Check sheet for the modelled part. Datum: model origin and axes. Units: mm. A direction names the side the tool comes from. Coordinates: 2 decimals unless noted, no trailing zeros. Loops run counter-clockwise (first coordinate to the right, second up) from the corner with the lowest first, then second, coordinate; pieces in that order, holes last.
Autodesk Inventor part; units mm, degrees
ref_plane "YZ Plane" through (0, 0, 0) normal (1, 0, 0) x (0, 1, 0)
ref_plane "XZ Plane" through (0, 0, 0) normal (0, 1, 0) x (-1, 0, 0)
ref_plane "XY Plane" through (0, 0, 0) normal (0, 0, 1) x (1, 0, 0)
sketch "Sketch1" plane through (0, 0, 0) normal (0, 1, 0) x (-1, 0, 0)
  circle A0 centre (0, 0) radius 4
  circle A1 centre (0, 0) radius 2.9
  dimension "d0" = 8
  dimension "d1" = 5.8
extrude "Extrusion1" add sketch "Sketch1" against normal blind 2 contours A0 | A1
extrude "Extrusion2" add sketch "Sketch1" along normal blind 6 contours A1
fillet "Fillet1" radius 1 1 edges at (2.9, 6, 0)
properties part number "Button_3DPrint"
(1) Section check A-A, the plane z = 0. Enter the section's corners in (x, y), plus the area to 3 significant figures.
(2) Section check B-B, the plane x = 0. Enter the section's corners in (y, z), plus the area to 3 significant figures.
(3) Section check D-D, the plane y = 0.5. Enter the section's corners in (x, z), plus the area to 3 significant figures.
(4) Gauge pin test, flat ends, axial feed: P1, Ø1, axis at y = 3, z = 1, coming from the +X side; P2, Ø1, axis at y = 4.5, z = -0.5, coming from the -X side; P3, Ø2, axis at x = 2.5, y = 4.5, coming from the -Z side. Record the tip position at first contact, or that the pin passes through.
(5) Scan lines: line 1 along Y through (x, z) = (1.5, 2.75); line 2 along X through (y, z) = (4, -2.5); line 3 along X through (y, z) = (0.75, -1.5). Record each from-to range of solid material in increasing order.
(6) Section check C-C, the plane y = -1.5. Enter the section's corners in (x, z), plus the area to 3 significant figures.
(7) Set-up check for faces 1 (the face through (0.867, -0.986, -3.905)), 2 (the face through (-3, 0, 1)): record each of +Z, -Z, +X, -X, +Y, -Y from which the full face is reachable in a straight line by a thin tool's end or side.
Determined:
1. outline: (-4, -2) - (4, -2) - (4, 0) - (2.9, 0) - (2.9, 5) arc R1 ccw to (1.9, 6) - (-1.9, 6) arc R1 ccw to (-2.9, 5) - (-2.9, 0) - (-4, 0) - close
1. area: 50.4 mm2
2. outline: (-2, -4) - (0, -4) - (0, -2.9) - (5, -2.9) arc R1 ccw to (6, -1.9) - (6, 1.9) arc R1 ccw to (5, 2.9) - (0, 2.9) - (0, 4) - (-2, 4) - close
2. area: 50.4 mm2
3. outline: circle Ø5.8 at (0, 0)
3. area: 26.4 mm2
4. P1: stops at x = 2.86
4. P2: stops at x = -2.9
4. P3: stops at z = -2.48
5. line 1: y = -2 to 0
5. line 2: x = -1.47 to 1.47
5. line 3: x = -2.48 to 2.48
6. outline: circle Ø8 at (0, 0)
6. area: 50.3 mm2
7. face 1: +Y, -Y
7. face 2: +Y
